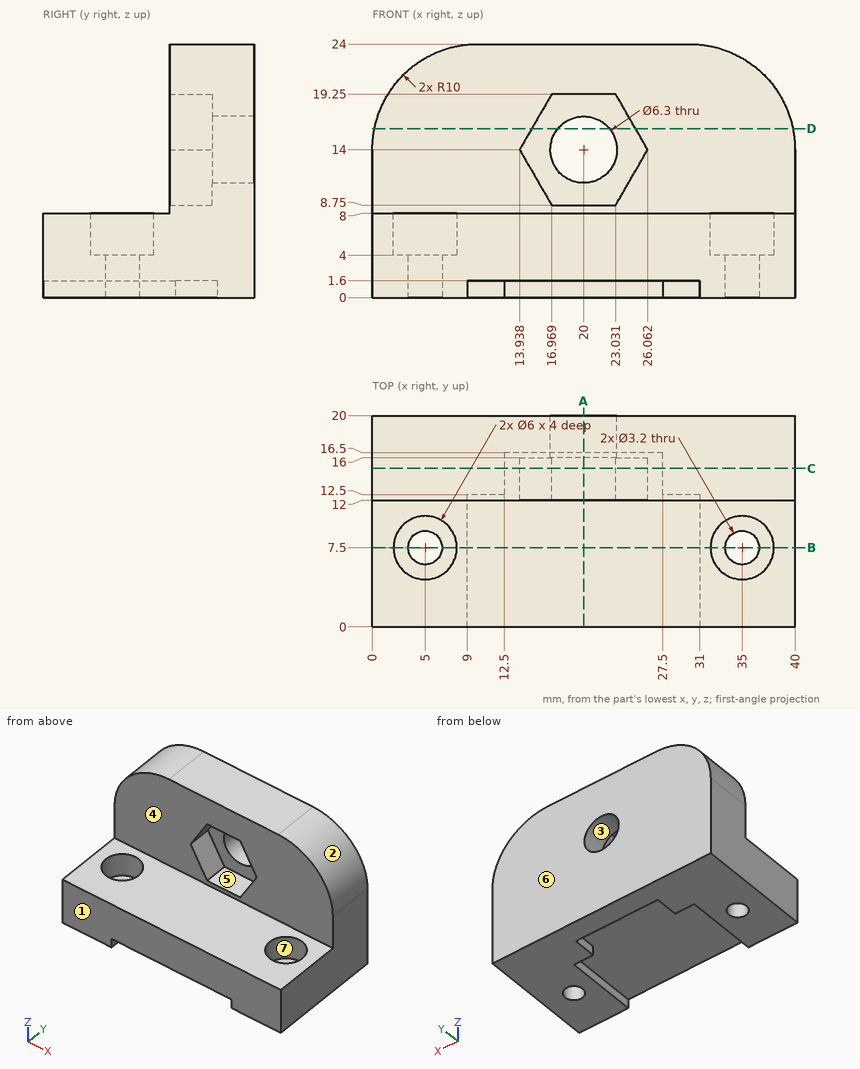
Here's the drawing with two shaded views (mm, measured from the low corner). I have some questions. A direction names the side the tool comes from. Round coordinates to 2 decimals unless told otherwise and drop trailing zeros. Loops run counter-clockwise (first coordinate to the right, second up) from the corner with the lowest first, then second, coordinate; pieces in that order, holes last. Notation, with made-up numbers: (25, 20) - (43, 20) arc R12 ccw to (43, 31) - close; hole circle Ø11 at (3.25, 63). An arc over 180 degrees is marked (long way). Use CSV: the item, a comma, the result in double quotes.
Item 1: If we mould it in two halves opening along Z, with no side actions, what happens to the marked faces 1, 2 and 3? For each: pulls with the +Z half, pulls with the -Z half, needs draft (parallel to the pull), parting line crosses it, or undercut.
Here are the results:
face 1,"needs draft"
face 2,"pulls with the +Z half"
face 3,"undercut"
Item 2: If we section it at C-C on y = 15: List the corners of the cut face in (x, z) for me, then the cut area to 3 significant figures.
Here are the results:
outline,"(0, 0) - (12.5, 0) - (12.5, 1.6) - (27.5, 1.6) - (27.5, 0) - (40, 0) - (40, 14) arc R10 ccw to (30, 24) - (10, 24) arc R10 ccw to (0, 14) - close; hole (13.94, 14) - (16.97, 8.75) - (23.03, 8.75) - (26.06, 14) - (23.03, 19.25) - (16.97, 19.25) - close"
area,"798 mm²"
Item 3: Will these pins go through, and if not, where does the flat tip stop? pin 1 (6 mm diameter, centred on x = 26.5, y = 4, fed in from +Z); pin 2 (5 mm diameter, centred on x = 19, z = 13, fed in from -Y); pin 3 (5 mm diameter, centred on x = 17, y = 5, fed in from -Z); pin 4 (0.5 mm diameter, centred on y = 6, z = 1, fed in from -X).
Here are the results:
pin 1,"stops at z = 8"
pin 2,"stops at y = 16"
pin 3,"stops at z = 1.6"
pin 4,"stops at x = 0"
Item 4: I need wall thicknesses on L1, parallel to Z at x = 22, y = 12.5; L2, parallel to Y at x = 35, z = 2.8; L3, parallel to Y at x = 5, z = 5.9. Which ranges of each line are inside material? Lowest first, please. Write a range as [from, to].
Here are the results:
L1,"z = [1.6, 8.75], [19.25, 24]"
L2,"y = [0, 5.9], [9.1, 20]"
L3,"y = [0, 4.5], [10.5, 20]"
Item 5: If we section it at A-A on x = 20: List the corners of the cut face in (y, z) for me, then the cut area to 3 significant figures.
Here are the results:
outline,"(0, 1.6) - (16.5, 1.6) - (16.5, 0) - (20, 0) - (20, 10.85) - (16, 10.85) - (16, 8.75) - (12, 8.75) - (12, 8) - (0, 8) - close; (12, 19.25) - (16, 19.25) - (16, 17.15) - (20, 17.15) - (20, 24) - (12, 24) - close"
area,"194 mm²"
Item 6: For the marked faces 4, 5, 6 and 7, which set-ups out of +Z, -Z, +X, -X, +Y, -Y let a thin tool reach every point of the face, with its end or its side?
Here are the results:
face 4,"+Z, +X, -X, -Y"
face 5,"-Y"
face 6,"+Z, -Z, +X, -X, +Y"
face 7,"+Z"
Item 7: If we section it at D-D on z = 16: List the corners of the cut face in (x, y) for me.
Here are the results:
outline,"(0.2, 12) - (15.09, 12) - (15.09, 16) - (17.57, 16) - (17.57, 20) - (0.2, 20) - close; (22.43, 16) - (24.91, 16) - (24.91, 12) - (39.8, 12) - (39.8, 20) - (22.43, 20) - close"
Item 8: If we section it at B-B on y = 7.5: List the corners of the cut face in (x, z) for me.
Here are the results:
outline,"(0, 0) - (3.4, 0) - (3.4, 4) - (2, 4) - (2, 8) - (0, 8) - close; (6.6, 0) - (9, 0) - (9, 1.6) - (31, 1.6) - (31, 0) - (33.4, 0) - (33.4, 4) - (32, 4) - (32, 8) - (8, 8) - (8, 4) - (6.6, 4) - close; (36.6, 0) - (40, 0) - (40, 8) - (38, 8) - (38, 4) - (36.6, 4) - close"
